Source: CAD feature listing. Evaluate the final solid. Frame: model axes, mm. Face numbers are marked on the shaded views. A direction names the side the tool comes from. Give positions to 0.01 mm unless a question says otherwise; leave off trailing zeros. Order: outer loops, then holes, each group sorted by start corner. A loop starts at its lowest first (then second) coordinate and runs counter-clockwise, first axis right, second up.
1) Section C-C, the plane z = 9. Return loops of the section in (x, y), plus the area to 3 significant figures.
2) Access query for the marked faces 1 and 2. Directions: +Z, -Z, +X, -X, +Y, -Y. A direction counts if a zero-diameter tool reaches every point of the face in a straight line with its end or side. Return the directions, or none.
3) Section B-B, the plane x = -10. Return loops of the section in (y, z).
4) First-contact query: P1, Ø4, axis at x = 32.639, z = 40.132, coming from the +Y side; P2, Ø5, axis at x = -32.639, z = 40.132, coming from the -Y side; P3, Ø4, axis at x = -22, z = 30, coming from the +Y side. Flat tips, straight axial feed; report the tip coordinate or a pass-through.
5) Section A-A, the plane y = 4.75. Return loops of the section in (x, z), plus the area to 3 significant figures.
6) Material intervals for line 1 (Z direction, x = -22, y = 6); line 2 (Y direction, x = -32, z = -3), sorted ascending.
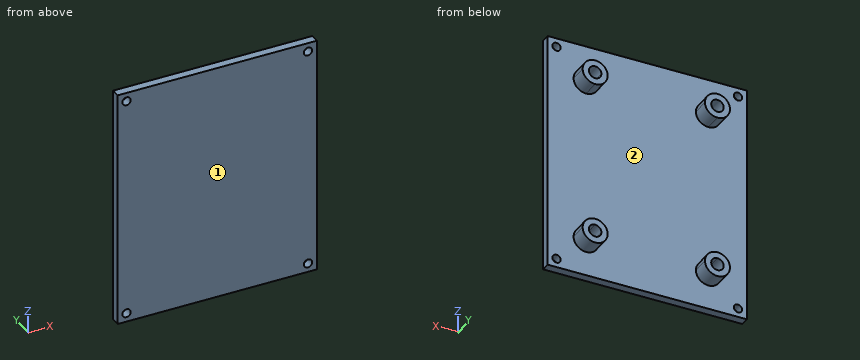
```python
from build123d import *

# Parameters (mm, degrees)
SKETCH2_W                                  = 71.628
SKETCH2_H                                  = 86.614
BOSS_EXTRUDE1_DEPTH                        = 1.5875
SKETCH3_R                                  = 1.5
CUT_EXTRUDE1_DEPTH                         = 3.175
MIRROR1_AT_THE_SECOND_PLANE_COPY_1_SKETC_R = 1.5
MIRROR1_AT_THE_SECOND_PLANE_COPY_1_DEPTH   = 3.175
BOSS_EXTRUDE2_DEPTH                        = 6.35
BOSS_EXTRUDE3_DEPTH                        = 0.549999916


with BuildPart() as part:
    # Sketch2 → Boss-Extrude1 (new body, symmetric)
    with BuildSketch(Plane(origin=(0, 0, 0), x_dir=(1, 0, 0), z_dir=(0, 1, 0))):
        Rectangle(SKETCH2_W, SKETCH2_H)
    extrude(amount=BOSS_EXTRUDE1_DEPTH, both=True)

    # Sketch3 → Cut-Extrude1 (cut)
    with BuildSketch(Plane(origin=(0, 1.5875, 0), x_dir=(1, 0, 0), z_dir=(0, 1, 0))):
        with Locations((-32.639, 40.132)):
            Circle(SKETCH3_R)
    cut_extrude1 = extrude(amount=-CUT_EXTRUDE1_DEPTH, mode=Mode.SUBTRACT)

    # Mirror1: Cut-Extrude1 across plane
    add(cut_extrude1.mirror(Plane(origin=(0, 0, 0), x_dir=(0, 0, 1), z_dir=(1, 0, 0))), mode=Mode.SUBTRACT)

    # Mirror1 at the second plane: Cut-Extrude1 across plane
    add(cut_extrude1.mirror(Plane.XY), mode=Mode.SUBTRACT)

    # Mirror1 at the second plane copy 1 sketc → Mirror1 at the second plane copy 1 (cut)
    with BuildSketch(Plane(origin=(0, 1.5875, 0), x_dir=(-1, 0, 0), z_dir=(0, 1, 0))):
        with Locations((-32.639, 40.132)):
            Circle(MIRROR1_AT_THE_SECOND_PLANE_COPY_1_SKETC_R)
    extrude(amount=-MIRROR1_AT_THE_SECOND_PLANE_COPY_1_DEPTH, mode=Mode.SUBTRACT)

    # Sketch4 → Boss-Extrude2 (add)
    with BuildSketch(Plane(origin=(0, 1.5875, 0), x_dir=(1, 0, 0), z_dir=(0, 1, 0))):
        with BuildLine():
            ThreePointArc((-22, 27.7500045), (-23.590987076, 31.590987076), (-19.7500045, 30))
            Line((-19.7500045, 30), (-17.499999983, 30))
            ThreePointArc((-17.499999983, 30), (-25.181980527, 33.181980527), (-22, 25.499999983))
            Line((-22, 25.499999983), (-22, 27.7500045))
        make_face()
        with BuildLine():
            Line((-17.499999983, 30), (-19.7500045, 30))
            ThreePointArc((-19.7500045, 30), (-20.409012924, 28.409012924), (-22, 27.7500045))
            Line((-22, 27.7500045), (-22, 25.499999983))
            ThreePointArc((-22, 25.499999983), (-18.818019473, 26.818019473), (-17.499999983, 30))
        make_face()
        with BuildLine():
            ThreePointArc((26.500000017, 30), (22, 34.500000017), (17.499999983, 30))
            Line((17.499999983, 30), (19.7500045, 30))
            ThreePointArc((19.7500045, 30), (22, 32.2499955), (24.2499955, 30))
            ThreePointArc((24.2499955, 30), (23.590987076, 28.409012924), (22, 27.7500045))
            Line((22, 27.7500045), (22, 25.499999983))
            ThreePointArc((22, 25.499999983), (25.181980527, 26.818019473), (26.500000017, 30))
        make_face()
        with BuildLine():
            Line((19.7500045, 30), (17.499999983, 30))
            ThreePointArc((17.499999983, 30), (18.818019473, 26.818019473), (22, 25.499999983))
            Line((22, 25.499999983), (22, 27.7500045))
            ThreePointArc((22, 27.7500045), (20.409012924, 28.409012924), (19.7500045, 30))
        make_face()
        with BuildLine():
            ThreePointArc((26.500000017, -30), (25.181980527, -26.818019473), (22, -25.499999983))
            Line((22, -25.499999983), (22, -27.7500045))
            ThreePointArc((22, -27.7500045), (23.590987076, -28.409012924), (24.2499955, -30))
            ThreePointArc((24.2499955, -30), (22, -32.2499955), (19.7500045, -30))
            Line((19.7500045, -30), (17.499999983, -30))
            ThreePointArc((17.499999983, -30), (22, -34.500000017), (26.500000017, -30))
        make_face()
        with BuildLine():
            Line((22, -27.7500045), (22, -25.499999983))
            ThreePointArc((22, -25.499999983), (18.818019473, -26.818019473), (17.499999983, -30))
            Line((17.499999983, -30), (19.7500045, -30))
            ThreePointArc((19.7500045, -30), (20.409012924, -28.409012924), (22, -27.7500045))
        make_face()
        with BuildLine():
            ThreePointArc((-17.499999983, -30), (-18.818019473, -26.818019473), (-22, -25.499999983))
            Line((-22, -25.499999983), (-22, -27.7500045))
            ThreePointArc((-22, -27.7500045), (-20.409012924, -28.409012924), (-19.7500045, -30))
            Line((-19.7500045, -30), (-17.499999983, -30))
        make_face()
        with BuildLine():
            Line((-22, -27.7500045), (-22, -25.499999983))
            ThreePointArc((-22, -25.499999983), (-25.181980527, -33.181980527), (-17.499999983, -30))
            Line((-17.499999983, -30), (-19.7500045, -30))
            ThreePointArc((-19.7500045, -30), (-23.590987076, -31.590987076), (-22, -27.7500045))
        make_face()
    extrude(amount=BOSS_EXTRUDE2_DEPTH)

    # Sketch4_3 → Boss-Extrude3 (add)
    with BuildSketch(Plane(origin=(0, 1.5875, 0), x_dir=(1, 0, 0), z_dir=(0, 1, 0))):
        with BuildLine():
            Line((-22, 27.7500045), (-22, 30))
            Line((-22, 30), (-19.7500045, 30))
            ThreePointArc((-19.7500045, 30), (-23.590987076, 31.590987076), (-22, 27.7500045))
        make_face()
        with BuildLine():
            Line((-19.7500045, 30), (-22, 30))
            Line((-22, 30), (-22, 27.7500045))
            ThreePointArc((-22, 27.7500045), (-20.409012924, 28.409012924), (-19.7500045, 30))
        make_face()
        with BuildLine():
            ThreePointArc((24.2499955, 30), (22, 32.2499955), (19.7500045, 30))
            Line((19.7500045, 30), (22, 30))
            Line((22, 30), (22, 27.7500045))
            ThreePointArc((22, 27.7500045), (23.590987076, 28.409012924), (24.2499955, 30))
        make_face()
        with BuildLine():
            Line((22, 30), (19.7500045, 30))
            ThreePointArc((19.7500045, 30), (20.409012924, 28.409012924), (22, 27.7500045))
            Line((22, 27.7500045), (22, 30))
        make_face()
        with BuildLine():
            ThreePointArc((24.2499955, -30), (23.590987076, -28.409012924), (22, -27.7500045))
            Line((22, -27.7500045), (22, -30))
            Line((22, -30), (19.7500045, -30))
            ThreePointArc((19.7500045, -30), (22, -32.2499955), (24.2499955, -30))
        make_face()
        with BuildLine():
            Line((22, -30), (22, -27.7500045))
            ThreePointArc((22, -27.7500045), (20.409012924, -28.409012924), (19.7500045, -30))
            Line((19.7500045, -30), (22, -30))
        make_face()
        with BuildLine():
            ThreePointArc((-19.7500045, -30), (-20.409012924, -28.409012924), (-22, -27.7500045))
            Line((-22, -27.7500045), (-22, -30))
            Line((-22, -30), (-19.7500045, -30))
        make_face()
        with BuildLine():
            Line((-22, -30), (-22, -27.7500045))
            ThreePointArc((-22, -27.7500045), (-23.590987076, -31.590987076), (-19.7500045, -30))
            Line((-19.7500045, -30), (-22, -30))
        make_face()
    extrude(amount=BOSS_EXTRUDE3_DEPTH)


solid = part.part
```
From the geometry:
1. outline: (-35.81, -1.59) - (35.81, -1.59) - (35.81, 1.59) - (-35.81, 1.59) - close
1. area: 227 mm2
2. face 1: +Z, -Z, +X, -X, -Y
2. face 2: +Y
3. outline: (-1.59, -43.31) - (1.59, -43.31) - (1.59, 43.31) - (-1.59, 43.31) - close
4. P1: stops at y = 1.59
4. P2: stops at y = -1.59
4. P3: stops at y = 2.14
5. outline: circle Ø9 at (-22, -30); circle Ø9 at (-22, 30); circle Ø9 at (22, -30); circle Ø9 at (22, 30); hole circle Ø4.5 at (-22, -30); hole circle Ø4.5 at (-22, 30); hole circle Ø4.5 at (22, -30); hole circle Ø4.5 at (22, 30)
5. area: 191 mm2
6. line 1: z = -34.5 to -32.25, -27.75 to -25.5, 25.5 to 27.75, 32.25 to 34.5
6. line 2: y = -1.59 to 1.59
